from build123d import *

# Parameters (mm, degrees)
F0_R     = 5
F1_DEPTH = 15
F3_DEPTH = 25


with BuildPart() as f1:
    # F0 (on Front) → F1 (new body)
    with BuildSketch(Plane.XZ):
        Polygon((-9.226497, -50.236377), (7.332118, -50.236377), (15, -41.6029), (15, 9.763623), (7.147167, 29.763623), (-6.655383, 29.763623), (-15, 9.963766), (-15, -40.236377), align=None)
        with BuildLine():
            Line((-4.617641, -35.236377), (-4.617641, -10.236377))
            ThreePointArc((-4.617641, -10.236377), (0.135772, -5.482964), (4.889185, -10.236377))
            Line((4.889185, -10.236377), (4.889185, -35.236377))
            ThreePointArc((4.889185, -35.236377), (0.135772, -39.98979), (-4.617641, -35.236377))
        make_face(mode=Mode.SUBTRACT)
        with Locations((0, 14.763623)):
            Circle(F0_R, mode=Mode.SUBTRACT)
    extrude(amount=F1_DEPTH)

    # F2 (on Right) → F3 (cut, symmetric)
    with BuildSketch(Plane.YZ):
        Polygon((-15, 9.763623), (-15, 5.763623), (-10, 5.763623), (-10, 39.44074), (-15, 39.44074), align=None)
    extrude(amount=F3_DEPTH, both=True, mode=Mode.SUBTRACT)


solid = f1.part
Part model, mm, in its own coordinate system. A direction names the side the tool comes from. Give positions to 0.01 mm unless a question says otherwise; leave off trailing zeros. Loops run counter-clockwise (first coordinate to the right, second up) from the corner with the lowest first, then second, coordinate; pieces in that order, holes last. Notation, with made-up numbers: (58.5, 22) -> (86.5, 22) arc R16 ccw to (86.5, 42) -> close; hole circle Ø4 at (49, -35). An arc over 180 degrees is marked (long way). Write each question's results on one line, items separated by ' | '. Start each with the question number.
Q1. Band-saw the part on B-B on z = -15. List the corners of the cut face in (x, y).
Q2. Band-saw the part on C-C on x = 0. List the corners of the cut face in (y, z), plus the area to 3 significant figures.
Q3. Which spindle directions (+Z, -Z, +X, -X, +Y, -Y) get a long thin tool onto all of the face, cutting with end or side? Do faces 1 (the face through (0, -10, 20)), 2 (the face through (0.031, -7.395, -5.484)), 3 (the face through (-12.15, -7.4, -45.17)). Say none if no direction does.
Q4. Wall check: L1, parallel to Z at x = 0, y = -4.75; L2, parallel to X at y = -8.25, z = -21.5; L3, parallel to Z at x = 4.5, y = -5.5. Give the ranges that are in metal, low to high.
Q5. Band-saw the part on D-D on y = -8.5. List the corners of the cut face in (x, z), plus the area to 3 significant figures.
Q6. Pull direction Z, two halves, no side cores. Call faces 4 (the face through (4.889, -7, -23)), 5 (the face through (-7, 0, -10)), 6 (the face through (11.13, -4.93, 19.62)), 7 (the face through (-1, -7, -50.236)): +Z half, -Z half, draft (parallel to the pull), parting line (faces both ways), or undercut.
Q7. Band-saw the part on A-A on y = -13.5. List the corners of the cut face in (x, z).
Q8. Pin check, flat tips, straight feed: P1, Ø5, axis at x = 10, y = -4.5, coming from the -Z side; P2, Ø1.5, axis at x = 7.5, y = -12, coming from the +Z side; P3, Ø7, axis at x = 4.5, z = 23.5, coming from the -Y side. Stop position of each tip, or through.
Results are:
1) outline: (-15, -15) -> (-4.62, -15) -> (-4.62, 0) -> (-15, 0) -> close; (4.89, -15) -> (15, -15) -> (15, 0) -> (4.89, 0) -> close
2) outline: (-15, -50.24) -> (0, -50.24) -> (0, -39.99) -> (-15, -39.99) -> close; (-15, -5.48) -> (0, -5.48) -> (0, 9.76) -> (-10, 9.76) -> (-10, 5.76) -> (-15, 5.76) -> close; (-10, 19.76) -> (0, 19.76) -> (0, 29.76) -> (-10, 29.76) -> close | area: 462 mm²
3) face 1: +Z, +X, -X, -Y | face 2: +Y, -Y | face 3: -Z, -X, +Y, -Y
4) L1: z = -50.24 to -39.99, -5.48 to 9.76, 19.76 to 29.76 | L2: x = -15 to -4.62, 4.89 to 15 | L3: z = -50.24 to -37.12, -8.35 to 12.58, 16.94 to 29.76
5) outline: (-15, -40.24) -> (-9.23, -50.24) -> (7.33, -50.24) -> (15, -41.6) -> (15, 9.76) -> (7.15, 29.76) -> (-6.66, 29.76) -> (-15, 9.96) -> close; hole circle Ø10 at (0, 14.76); hole (-4.62, -35.24) arc R4.75 ccw to (4.89, -35.24) -> (4.89, -10.24) arc R4.75 ccw to (-4.62, -10.24) -> close | area: 1,790 mm²
6) face 4: undercut | face 5: draft | face 6: +Z half | face 7: -Z half
7) outline: (-15, -40.24) -> (-9.23, -50.24) -> (7.33, -50.24) -> (15, -41.6) -> (15, 5.76) -> (-15, 5.76) -> close; hole (-4.62, -35.24) arc R4.75 ccw to (4.89, -35.24) -> (4.89, -10.24) arc R4.75 ccw to (-4.62, -10.24) -> close
8) P1: stops at z = -50.05 | P2: stops at z = 5.76 | P3: stops at y = -10
